Can you work these out from the drawing? Everything is in mm from the part's minimum corner. Round coordinates to 2 decimals unless told otherwise and drop trailing zeros. Order: outer loops, then holes, each group sorted by start corner. A loop starts at its lowest first (then second) coordinate and runs counter-clockwise, first axis right, second up. Notation, with made-up numbers: M 55.25,65.25 L 105.25,65.25 A8 ccw 105.25,77.25 Z; hole C 12,-34.75 d5. An arc over 180 degrees is marked long. Answer as CSV lines item,"result". Start each with the question number.
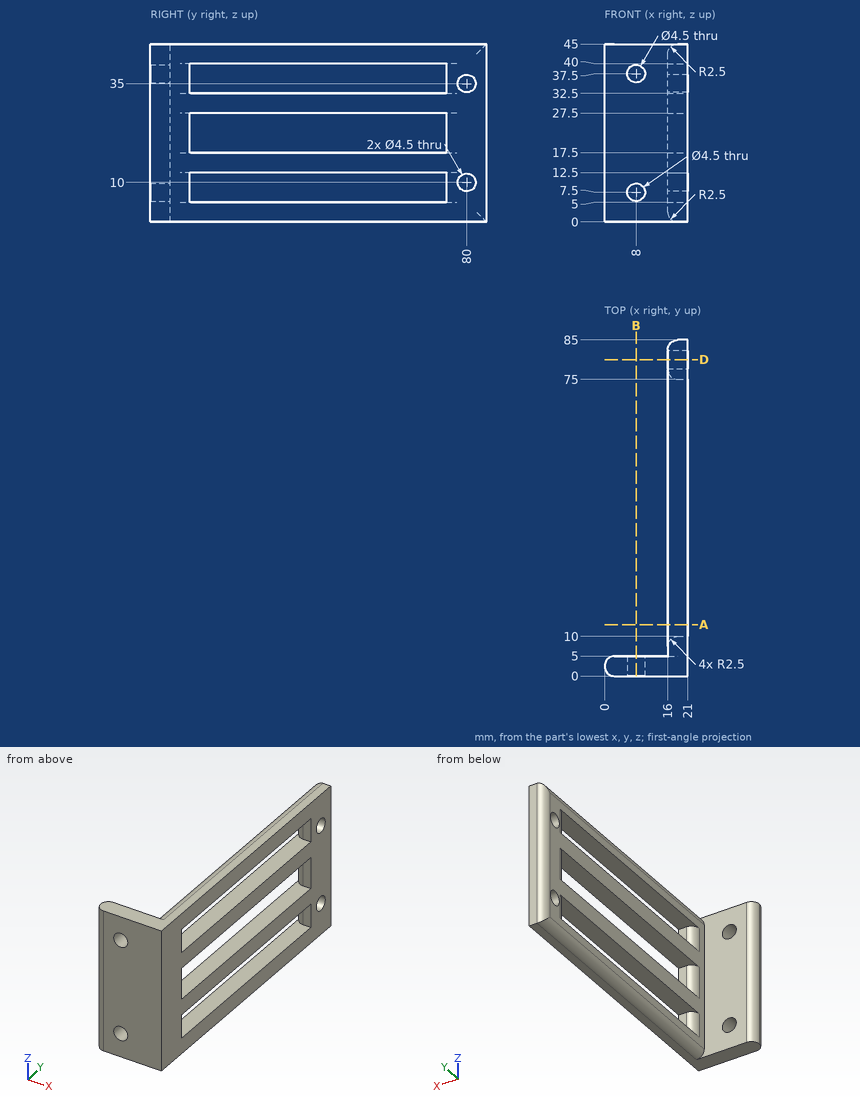
(1) If I drill on line 1 along Z through (x, y) = (18.4, 80); line 2 along Z through (x, y) = (8, 1.2); line 3 along X through (y, z) = (48, 13), over which ranges is the centre line in solid material (lowest first)?
(2) I want a section at A-A on y = 13. Write out the boundary of the cut face in (x, z).
(3) I want a section at D-D on y = 80. Write out the boundary of the cut face in (x, z), and give its area (3 significant figures).
(4) I want a section at B-B on x = 8. Write out the boundary of the cut face in (y, z).
(5) I'm going to push flat-ended pins straight in: P1, Ø5, axis at y = 80, z = 10, coming from the -X side; P2, Ø1.5, axis at x = 17.5, y = 15.5, coming from the -Z side. Where does each tip first touch, or does it pass through?
From the geometry:
1,line 1,"0 to 7.75, 12.25 to 32.75, 37.25 to 45"
1,line 2,"0 to 5.25, 9.75 to 35.25, 39.75 to 45"
1,line 3,"16 to 21"
2,outline,"M 16,2.5 A2.5 ccw 18.5,0 L 21,0 L 21,5 L 16,5 Z; M 16,12.5 L 21,12.5 L 21,17.5 L 16,17.5 Z; M 16,27.5 L 21,27.5 L 21,32.5 L 16,32.5 Z; M 16,40 L 21,40 L 21,45 L 18.5,45 A2.5 ccw 16,42.5 Z"
3,outline,"M 16,2.5 A2.5 ccw 18.5,0 L 21,0 L 21,7.75 L 16,7.75 Z; M 16,12.25 L 21,12.25 L 21,32.75 L 16,32.75 Z; M 16,37.25 L 21,37.25 L 21,45 L 18.5,45 A2.5 ccw 16,42.5 Z"
3,area,"177 mm²"
4,outline,"M 0,0 L 5,0 L 5,5.25 L 0,5.25 Z; M 0,9.75 L 5,9.75 L 5,35.25 L 0,35.25 Z; M 0,39.75 L 5,39.75 L 5,45 L 0,45 Z"
5,P1,"x = 16"
5,P2,"z = 0.01"
